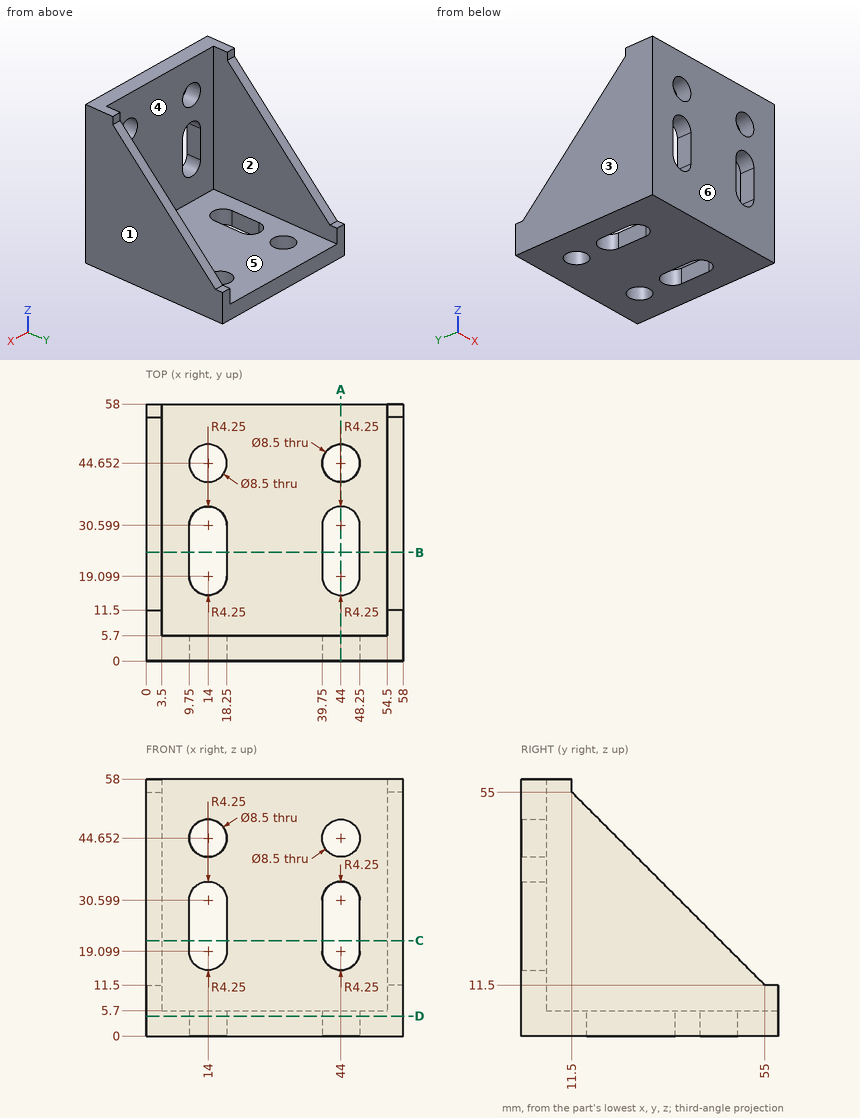
Geometry check sheet. Reference: drawing and pictorial views, mm from the part's lowest x, y, z. A direction names the side the tool comes from. Round coordinates to 2 decimals unless told otherwise and drop trailing zeros. Loops run counter-clockwise (first coordinate to the right, second up) from the corner with the lowest first, then second, coordinate; pieces in that order, holes last.
1. Sectioned sample at B-B on y = 24.5. Record the boundary of the cut face in (x, z).
2. Scan lines: probe 1 along Y at (x, z) = (14, 2.15); probe 2 along X at (y, z) = (12.5, 24.5). Record each from-to range of solid material in increasing order.
3. Sectioned sample at D-D on z = 4.5. Record the boundary of the cut face in (x, y).
4. Set-up check for the marked faces 5 and 6: record each of +Z, -Z, +X, -X, +Y, -Y from which the full face is reachable in a straight line by a thin tool's end or side.
5. Gauge pin test, flat ends, axial feed: pin 1 Ø2.5 at (x, y) = (2.5, 57) entering from +Z; pin 2 Ø7.5 at (x, z) = (14, 44.65) entering from +Y; pin 3 Ø15.5 at (x, z) = (20, 32.5) entering from +Y; pin 4 Ø3 at (x, y) = (40, 32.5) entering from +Z. Record the tip position at first contact, or that the pin passes through.
6. Sectioned sample at C-C on z = 21.5. Record the boundary of the cut face in (x, y), and give its area (3 significant figures).
7. Sectioned sample at A-A on x = 44. Record the boundary of the cut face in (y, z).
8. Mould release check, pull along X, two halves, no side actions. Record for the marked faces 1, 2, 3 and 4: released by +X, released by -X, zero draft, split by the parting line, or undercut.
Recorded:
1. outline: (0, 0) - (9.75, 0) - (9.75, 5.7) - (3.5, 5.7) - (3.5, 42) - (0, 42) - close; (18.25, 0) - (39.75, 0) - (39.75, 5.7) - (18.25, 5.7) - close; (48.25, 0) - (58, 0) - (58, 42) - (54.5, 42) - (54.5, 5.7) - (48.25, 5.7) - close
2. probe 1: y = 0 to 14.85, 34.85 to 40.4, 48.9 to 58
2. probe 2: x = 0 to 3.5, 54.5 to 58
3. outline: (0, 0) - (58, 0) - (58, 58) - (0, 58) - close; hole (9.75, 19.1) arc R4.25 ccw to (18.25, 19.1) - (18.25, 30.6) arc R4.25 ccw to (9.75, 30.6) - close; hole circle Ø8.5 at (14, 44.65); hole (39.75, 19.1) arc R4.25 ccw to (48.25, 19.1) - (48.25, 30.6) arc R4.25 ccw to (39.75, 30.6) - close; hole circle Ø8.5 at (44, 44.65)
4. face 5: +Z, +Y
4. face 6: +Z, -Z, +X, -X, -Y
5. pin 1: stops at z = 11.5
5. pin 2: passes through
5. pin 3: stops at y = 5.7
5. pin 4: stops at z = 5.7
6. outline: (0, 0) - (9.75, 0) - (9.75, 5.7) - (3.5, 5.7) - (3.5, 45) - (0, 45) - close; (18.25, 0) - (39.75, 0) - (39.75, 5.7) - (18.25, 5.7) - close; (48.25, 0) - (58, 0) - (58, 45) - (54.5, 45) - (54.5, 5.7) - (48.25, 5.7) - close
6. area: 509 mm2
7. outline: (0, 0) - (14.85, 0) - (14.85, 5.7) - (5.7, 5.7) - (5.7, 14.85) - (0, 14.85) - close; (0, 34.85) - (5.7, 34.85) - (5.7, 40.4) - (0, 40.4) - close; (0, 48.9) - (5.7, 48.9) - (5.7, 58) - (0, 58) - close; (34.85, 0) - (40.4, 0) - (40.4, 5.7) - (34.85, 5.7) - close; (48.9, 0) - (58, 0) - (58, 5.7) - (48.9, 5.7) - close
8. face 1: released by +X
8. face 2: undercut
8. face 3: released by -X
8. face 4: undercut
